Could you check a few things on this model? Use its own coordinates, in mm. A direction names the side the tool comes from. Coordinates: 2 decimals unless noted, no trailing zeros. Loops run counter-clockwise (first coordinate to the right, second up) from the corner with the lowest first, then second, coordinate; pieces in that order, holes last.
from build123d import *

# Parameters (mm, degrees)
CROQUIS1_W              = 54
CROQUIS1_H              = 20
SALIENTE_EXTRUIR1_DEPTH = 4
CROQUIS2_W              = 20
CROQUIS2_H              = 40
SALIENTE_EXTRUIR2_DEPTH = 6
CROQUIS3_R              = 10.02395417
SALIENTE_EXTRUIR3_DEPTH = 3.6
CROQUIS4_R              = 3
SALIENTE_EXTRUIR4_DEPTH = 5.5
CROQUIS5_W              = 20
CROQUIS5_H              = 40
SALIENTE_EXTRUIR5_DEPTH = 28.5


with BuildPart() as part:
    # Croquis1 → Saliente-Extruir1 (new body)
    with BuildSketch(Plane(origin=(0, 0, 0), x_dir=(0, 1, 0), z_dir=(0, 0, 1))):
        Rectangle(CROQUIS1_W, CROQUIS1_H)
    extrude(amount=SALIENTE_EXTRUIR1_DEPTH)

    # Croquis2 → Saliente-Extruir2 (add)
    with BuildSketch(Plane.XY.offset(4)):
        Rectangle(CROQUIS2_W, CROQUIS2_H)
    extrude(amount=SALIENTE_EXTRUIR2_DEPTH)

    # Croquis3 → Saliente-Extruir3 (add)
    with BuildSketch(Plane.XY.offset(10)):
        with Locations(Location((-0.116229886, 9.884437844, 0), (0, 0, 189.593450482))):
            Circle(CROQUIS3_R)
    extrude(amount=SALIENTE_EXTRUIR3_DEPTH)

    # Croquis4 → Saliente-Extruir4 (add)
    with BuildSketch(Plane.XY.offset(13.6)):
        with Locations((-0.116229886, 9.884437844)):
            Circle(CROQUIS4_R)
    extrude(amount=SALIENTE_EXTRUIR4_DEPTH)

    # Croquis5 → Saliente-Extruir5 (add)
    with BuildSketch(Plane(origin=(0, 0, 0), x_dir=(1, 0, 0), z_dir=(0, 0, -1))):
        Rectangle(CROQUIS5_W, CROQUIS5_H)
    extrude(amount=SALIENTE_EXTRUIR5_DEPTH)


solid = part.part
(1) Imagine slicing it at B-B, the plane x = 8. Write out the boundary of the cut face in (y, z), and give its area (3 significant figures).
Answers:
outline: (-27, 0) - (-20, 0) - (-20, -28.5) - (20, -28.5) - (20, 0) - (27, 0) - (27, 4) - (20, 4) - (20, 10) - (15.77, 10) - (15.77, 13.6) - (4, 13.6) - (4, 10) - (-20, 10) - (-20, 4) - (-27, 4) - close
area: 1,640 mm2
(2) Imagine slicing it at A-A, the plane y = 5. Write out the boundary of the cut face in (x, z).
Answers:
outline: (-10, -28.5) - (10, -28.5) - (10, 10) - (8.64, 10) - (8.64, 13.6) - (-8.87, 13.6) - (-8.87, 10) - (-10, 10) - close
(3) For pin 1 (3 mm diameter, centred on x = -7.5, z = -18, fed in from -Y); pin 2 (3.5 mm diameter, centred on x = -2, y = -22.5, fed in from +Z); pin 3 (10 mm diameter, centred on x = -6.5, y = 1, fed in from +Z); pin 4 (6.5 mm diameter, centred on x = -4, z = 6.5, fed in from -Y), each with a flat end and sliding along its axis, tell me the tip position at first contact or that it passes through.
Answers:
pin 1: stops at y = -20
pin 2: stops at z = 4
pin 3: stops at z = 13.6
pin 4: stops at y = -27
(4) Imagine slicing it at D-D, the plane x = 1.5. Write out the boundary of the cut face in (y, z).
Answers:
outline: (-27, 0) - (-20, 0) - (-20, -28.5) - (20, -28.5) - (20, 0) - (27, 0) - (27, 4) - (20, 4) - (20, 10) - (19.78, 10) - (19.78, 13.6) - (12.41, 13.6) - (12.41, 19.1) - (7.36, 19.1) - (7.36, 13.6) - (-0.01, 13.6) - (-0.01, 10) - (-20, 10) - (-20, 4) - (-27, 4) - close
(5) I need wall thicknesses on probe 1 along Y at (x, z) = (-4.25, -22); probe 2 along Z at (x, y) = (-2.75, 21.5); probe 3 along Z at (x, y) = (-3.5, -17). Which ranges of each line are inside material? Lowest first, please.
Answers:
probe 1: y = -20 to 20
probe 2: z = 0 to 4
probe 3: z = -28.5 to 10
(6) Imagine slicing it at C-C, the plane z = -3. Write out the boundary of the cut face in (x, y), and give its area (3 significant figures).
Answers:
outline: (-10, -20) - (10, -20) - (10, 20) - (-10, 20) - close
area: 800 mm2
(7) Which directions (+Z, -Z, +X, -X, +Y, -Y) give clear straight access to the entire face, cutting with the end or side of a thin tool? Please do faces 1 (the face through (0, 20, -14)), 2 (the face through (0, -24, 4)), 3 (the face through (0, -20, -14)), 4 (the face through (0.396, 19.895, 11.775)).
Answers:
face 1: -Z, +X, -X, +Y
face 2: +Z, +X, -X, -Y
face 3: -Z, +X, -X, -Y
face 4: +Z
